Autodesk Inventor part; units mm, degrees
ref_plane "YZ Plane" through (0, 0, 0) normal (1, 0, 0) x (0, 1, 0)
ref_plane "XZ Plane" through (0, 0, 0) normal (0, 1, 0) x (-1, 0, 0)
ref_plane "XY Plane" through (0, 0, 0) normal (0, 0, 1) x (1, 0, 0)
sketch "Sketch1" plane through (0, 0, 0) normal (0, 1, 0) x (-1, 0, 0)
  circle A0 centre (0, 0) radius 35
  dimension "d0" = 70
extrude "Extrusion1" add sketch "Sketch1" along normal blind 700
sketch "Sketch2" plane through (0, 700, 0) normal (0, 1, 0) x (1, 0, 0)
  line L0 (0, 0) -> (0, -35)
  line L1 (0, -35) -> (35, -35)
  line L2 (35, -35) -> (35, 35)
  line L3 (35, 35) -> (-35, 35)
  line L4 (-35, 35) -> (-35, -35)
  circle A0 centre (0, 0) radius 35
  line L5 (-35, -35) -> (0, -35)
  dimension "d3" = 35
  dimension "d4" = 35
  dimension "d5" = 70
  dimension "d6" = 70
  dimension "d7" = 70
extrude "Extrusion2" add sketch "Sketch2" along normal blind 70
sketch "Sketch3" plane through (-35, 700, 35) normal (0, 0, 1) x (1, 0, 0)
  circle A0 centre (35, 35) radius 25
  point P0 (35, -700)
  dimension "d10" = 50
extrude "Extrusion3" add sketch "Sketch3" along normal blind 300
sketch "Sketch4" plane through (35, 700, -35) normal (0, 0, -1) x (-1, 0, 0)
  line L0 (70, 70) -> (70, 35)
  line L1 (70, 0) -> (70, 70)
  line L2 (70, 35) -> (35, 35)
  circle A0 centre (35, 35) radius 25
  point P0 (35, -700)
  dimension "d13" = 35
  dimension "d14" = 35
  dimension "d15" = 50
extrude "Extrusion4" add sketch "Sketch4" along normal blind 300
fillet "Fillet1" radius 35 2 edges at (35, 770, 0) (-35, 770, 0)
thread "Thread1"
properties part number "fuso"
Here's how the part is built. I have some questions about the finished solid (model axes, mm). A direction names the side the tool comes from. Round coordinates to 2 decimals unless told otherwise and drop trailing zeros. Write each loop counter-clockwise with the first axis right and the second up, starting at its lowest first coordinate (ties: lowest second). Pieces come first, ordered by that corner, then holes. Notation, with made-up numbers: (-32, 80.25) -> (5, 80.25) arc R22 cw to (5, 95.25) -> close; hole circle Ø10 at (72.25, -23.75). An arc over 180 degrees is marked (long way). One line per item, written item: value.
1) Suppose I cut it at A-A on x = 10. List the corners of the cut face in (y, z) for me.
Filled sheet:
outline: (0, -33.54) -> (700, -33.54) -> (700, -35) -> (712.09, -35) -> (712.09, -335) -> (757.91, -335) -> (757.91, -35) -> (768.54, -35) -> (768.54, 35) -> (757.91, 35) -> (757.91, 335) -> (712.09, 335) -> (712.09, 35) -> (700, 35) -> (700, 33.54) -> (0, 33.54) -> close
2) If I drill on line 1 (Z direction, x = 0.5, y = 204); line 2 (Z direction, x = -31, y = 242); line 3 (Y direction, x = -8, z = -102.5), over which ranges is the centre line in solid material (lowest first)? Write a range as [from, to].
Filled sheet:
line 1: z = [-35, 35]
line 2: z = [-16.25, 16.25]
line 3: y = [711.31, 758.69]
3) I'm going to push flat-ended pins straight in: pin 1 Ø1 at (x, z) = (-10.5, 9) entering from +Y; pin 2 Ø4 at (x, y) = (0.5, 239.5) entering from +Z; pin 3 Ø1 at (x, z) = (-18.5, 89) entering from +Y. Where does each tip first touch, or does it pass through?
Filled sheet:
pin 1: stops at y = 768.54
pin 2: stops at z = 35
pin 3: stops at y = 752.35
4) Suppose I cut it at C-C on y = 573.5. List the corners of the cut face in (x, z) for me.
Filled sheet:
outline: circle Ø70 at (0, 0)
5) For faces 1 (the face through (28, 345, 21)), 2 (the face through (-28, 700, 26)), 3 (the face through (-8, 711, 35)), which set-ups out of +Z, -Z, +X, -X, +Y, -Y let a thin tool reach every point of the face, with its end or its side?
Filled sheet:
face 1: -Y
face 2: +Z, -X, -Y
face 3: +Z
6) We'd pull the mould along Y, two halves only. Please class faces 4 (the face through (-24.475, 760.02, 0.49)), 5 (the face through (11.5, 757.2, 182.9)), 6 (the face through (28, 700, 28)): released by +Y, released by -Y, zero draft, split by the parting line, or undercut.
Filled sheet:
face 4: released by +Y
face 5: split by the parting line
face 6: released by -Y
7) Suppose I cut it at D-D on z = -240. List the corners of the cut face in (x, y) for me.
Filled sheet:
outline: circle Ø50 at (0, 735)
